Verification items for the finished model (mm, model axes). Face numbers are marked on the shaded views. A direction names the side the tool comes from. Round coordinates to 2 decimals unless told otherwise and drop trailing zeros. Write each loop counter-clockwise with the first axis right and the second up, starting at its lowest first coordinate (ties: lowest second). Pieces come first, ordered by that corner, then holes.
from build123d import *

# Parameters (mm, degrees)
SKETCH1_R           = 9.5
BOSS_EXTRUDE1_DEPTH = 10
CHAMFER1_SIZE       = 2
SKETCH2_R           = 13
BOSS_EXTRUDE2_DEPTH = 3
BOSS_EXTRUDE3_DEPTH = 3.5
BOSS_EXTRUDE3_TAPER = 8
FILLET1_R           = 1
SKETCH3_W           = 2.3
SKETCH3_H           = 1.548065916
CUT_EXTRUDE1_DEPTH  = 1


with BuildPart() as part:
    # Sketch1 → Boss-Extrude1 (new body)
    with BuildSketch(Plane.XY):
        Circle(SKETCH1_R)
    extrude(amount=BOSS_EXTRUDE1_DEPTH)

    # Chamfer1
    chamfer1_edges = [part.edges().sort_by_distance(p)[0] for p in [
        (-9.5, 0, 0),
    ]]
    chamfer(chamfer1_edges, length=CHAMFER1_SIZE)

    # Sketch2 → Boss-Extrude2 (add)
    with BuildSketch(Plane.XY.offset(10)):
        Circle(SKETCH2_R)
    extrude(amount=BOSS_EXTRUDE2_DEPTH)

    # Sketch4 → Boss-Extrude3 (add)
    with BuildSketch(Plane.XY.offset(13)):
        with BuildLine():
            ThreePointArc((3, 10.583005244), (0, 11), (-3, 10.583005244))
            Line((-3, 10.583005244), (-3, 4))
            ThreePointArc((-3, 4), (0, 5), (3, 4))
            Line((3, 4), (3, 10.583005244))
        make_face()
        with BuildLine():
            ThreePointArc((3, -4), (0, -5), (-3, -4))
            Line((-3, -4), (-3, -10.583005244))
            ThreePointArc((-3, -10.583005244), (0, -11), (3, -10.583005244))
            Line((3, -10.583005244), (3, -4))
        make_face()
    extrude(amount=BOSS_EXTRUDE3_DEPTH, taper=BOSS_EXTRUDE3_TAPER)

    # Fillet1
    fillet1_edges = [part.edges().sort_by_distance(p)[0] for p in [
        (-13, 0, 10),
        (-13, 0, 13),
    ]]
    fillet(fillet1_edges, radius=FILLET1_R)

    # Sketch3 → Cut-Extrude1 (cut)
    with BuildSketch(Plane.XY.offset(13)):
        Polygon((-1.625120105, -2.013905208), (-1.625120105, 3.480258709), (1.874879895, 3.480258709), (1.874879895, -2.019741291), (1.274879895, -2.019741291), (1.274879895, 0.732192793), (-1.025120105, 0.732192793), (-1.025120105, -2.013905208), align=None)
        with Locations((0.124879895, 2.106225751)):
            Rectangle(SKETCH3_W, SKETCH3_H, mode=Mode.SUBTRACT)
        Polygon((5.374879895, 3.480258709), (8.874879895, 3.480258709), (8.874879895, 2.880258709), (5.974879895, 2.880258709), (5.974879895, 1.320855687), (8.874879895, 1.320855687), (8.874879895, -1.419741291), (8.874879895, -2.019741291), (5.374879895, -2.019741291), (5.374879895, -1.419741291), (8.274879895, -1.419741291), (8.274879895, 0.720855687), (5.374879895, 0.720855687), align=None)
        Polygon((-8.615536657, 3.480258709), (-8.615536657, -2.013905208), (-5.125120105, -2.013905208), (-5.125120105, 0.73317675), (-6.870328381, 0.73317675), (-6.870328381, 0.13317675), (-5.725120105, 0.13317675), (-5.725120105, -1.413905208), (-8.015536657, -1.413905208), (-8.015536657, 2.880258709), (-5.125120105, 2.880258709), (-5.125120105, 3.480258709), align=None)
    extrude(amount=-CUT_EXTRUDE1_DEPTH, mode=Mode.SUBTRACT)


solid = part.part
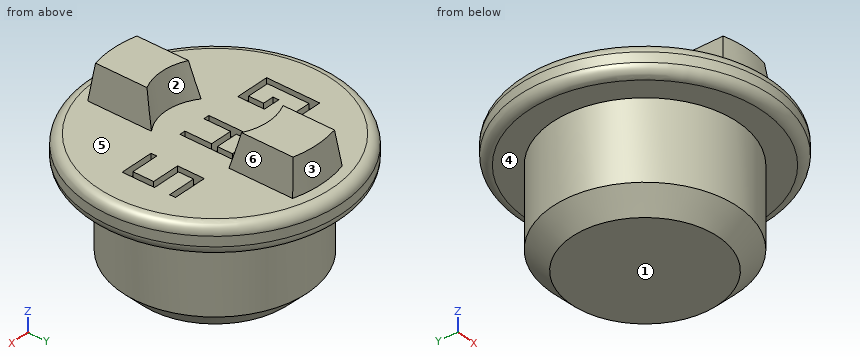
Q1. Material ranges on line 1 along X through (y, z) = (-7.75, 2.25); line 2 along Z through (x, y) = (-6, 2.75); line 3 along Y through (x, z) = (-0.25, 6), recorded low to high.
Recorded:
line 1: x = -5.49 to 5.49
line 2: z = 0 to 13
line 3: y = -9.5 to 9.5
Q2. Depth check by flat-ended pin: P1, Ø6, axis at y = -4, z = 6.5, coming from the -X side; P2, Ø0.5, axis at y = -0.5, z = 12.5, coming from the +X side; P3, Ø0.8, axis at x = 6.5, z = 12.5, coming from the -Y side. Enter the tip coordinate at first touch or a pass-through.
Recorded:
P1: stops at x = -9.45
P2: stops at x = 12.96
P3: stops at y = -11.4
Q3. Sectioned sample at C-C (z = 5.75). Enter the section's corners in (x, y), plus the area to 3 significant figures.
Recorded:
outline: circle Ø19 at (0, 0)
area: 284 mm2
Q4. Release check for a two-part mould opening along Y. For the marked faces 1, 2 and 3 record: released by +Y, released by -Y, zero draft, split by the parting line, or undercut.
Recorded:
face 1: zero draft
face 2: undercut
face 3: released by +Y
Q5. Sectioned sample at A-A (z = 13.5). Enter the section's corners in (x, y).
Recorded:
outline: (-2.93, -10.53) arc R10.93 ccw to (2.93, -10.53) - (2.93, -4.14) arc R5.07 cw to (-2.93, -4.14) - close; (-2.93, 4.14) arc R5.07 cw to (2.93, 4.14) - (2.93, 10.53) arc R10.93 ccw to (-2.93, 10.53) - close
Q6. Tool access check on the marked faces 4, 5 and 6. Record the directions out of +Z, -Z, +X, -X, +Y, -Y that give a thin tool (end or side, any length) a straight path to the whole face; none if there is none.
Recorded:
face 4: -Z
face 5: +Z
face 6: +Z, +X, +Y, -Y
